```python
from build123d import *

# Parameters (mm, degrees)
SKETCH7_W               = 7.9375
SKETCH7_H               = 3.000000096
BOSS_EXTRUDE2_DEPTH     = 130.175
SKETCH8_W               = 3.000000096
SKETCH8_H               = 7.9375
BOSS_EXTRUDE3_DEPTH     = 130.175
BOSS_EXTRUDE4_DEPTH     = 130.175
CUT_EXTRUDE4_DEPTH      = 2.515570892
CUT_EXTRUDE4_DEPTH_BACK = 11.4775001
CUT_EXTRUDE5_DEPTH      = 11.4775001
CUT_EXTRUDE5_DEPTH_BACK = 2.500000148


with BuildPart() as part:
    # Sketch7 → Boss-Extrude2 (new body, symmetric)
    with BuildSketch(Plane.XY):
        with Locations((-6.50875, -3.000000096)):
            Rectangle(SKETCH7_W, SKETCH7_H)
    extrude(amount=BOSS_EXTRUDE2_DEPTH, both=True)

    # Sketch8 → Boss-Extrude3 (add, symmetric)
    with BuildSketch(Plane.XY):
        with Locations((-3.000000096, -6.50875)):
            Rectangle(SKETCH8_W, SKETCH8_H)
    extrude(amount=BOSS_EXTRUDE3_DEPTH, both=True)

    # Sketch11 → Boss-Extrude4 (add, symmetric)
    with BuildSketch(Plane.XY):
        with BuildLine():
            Line((-2.54, 1.500000048), (-2.54, -1.500000048))
            Line((-2.54, -1.500000048), (-10.4775, -1.500000048))
            Line((-10.4775, -1.500000048), (-10.4775, -4.500000144))
            Line((-10.4775, -4.500000144), (-6.745064174, -4.500000144))
            Line((-6.745064174, -4.500000144), (-4.500000144, -6.745064174))
            Line((-4.500000144, -6.745064174), (-4.500000144, -10.4775))
            Line((-4.500000144, -10.4775), (-1.500000048, -10.4775))
            Line((-1.500000048, -10.4775), (-1.500000048, -2.54))
            Line((-1.500000048, -2.54), (1.500000048, -2.54))
            add(Edge.make_bspline(
                [(-2.54, 1.500000048), (-1.295649087, 1.635512934), (-0.042467258, 0.473225958), (1.297713539, -0.292226779), (1.263724591, -2.340394541), (1.500000048, -2.54)],
                knots=[0, 0, 0, 0, 0.496686972, 0.741346965, 0.899739924, 0.899739924, 0.899739924, 0.899739924], degree=3))
        make_face()
    extrude(amount=BOSS_EXTRUDE4_DEPTH, both=True)

    # Sketch14 → Cut-Extrude4 (cut, two sides)
    with BuildSketch(Plane(origin=(0, 0, 0), x_dir=(1, 0, 0), z_dir=(0, 1, 0))) as cut_extrude4_sk:
        Polygon((-10.4775, -116.5225), (-10.4775, -137.4775), (10.4775, -137.4775), align=None)
        Polygon((-10.4775, 116.5225), (10.4775, 137.4775), (-10.4775, 137.4775), align=None)
    extrude(amount=CUT_EXTRUDE4_DEPTH, mode=Mode.SUBTRACT)
    extrude(cut_extrude4_sk.sketch, amount=-CUT_EXTRUDE4_DEPTH_BACK, mode=Mode.SUBTRACT)

    # Sketch17 → Cut-Extrude5 (cut, two sides)
    with BuildSketch(Plane(origin=(0, 0, 0), x_dir=(0, -1, 0), z_dir=(-1, 0, 0))) as cut_extrude5_sk:
        Polygon((10.4775, 137.4775), (10.4775, 116.5225), (-10.4775, 137.4775), align=None)
        Polygon((10.4775, -116.5225), (-10.4775, -137.4775), (10.4775, -137.4775), align=None)
    extrude(amount=CUT_EXTRUDE5_DEPTH, mode=Mode.SUBTRACT)
    extrude(cut_extrude5_sk.sketch, amount=-CUT_EXTRUDE5_DEPTH_BACK, mode=Mode.SUBTRACT)


solid = part.part
```
The listing builds one solid part. Answer for the finished solid, in the listing's coordinates (mm). A direction names the side the tool comes from. Round coordinates to 2 decimals unless told otherwise and drop trailing zeros. Answer as a JSON object with one key per item and string values. Group by question number.
Q1. Each of these flat-tipped pins is pushed along its axis until it touches: pin 1 Ø4 at (y, z) = (-5.5, -5.5) entering from +X; pin 2 Ø2 at (x, z) = (-7, 46) entering from -Y; pin 3 Ø4 at (x, z) = (-5, -50.5) entering from +Y. Where does it stop, or does it pass through?
Q2. Straight lines are drawn through the part: line 1 along Y through (x, z) = (0.75, 7.5); line 2 along Y through (x, z) = (-8.5, -36); line 3 along X through (y, z) = (-2.5, 59). For each, find the intervals that lie inside material, in ascending order.
Q3. Which of the six approach directions +Z, -Z, +X, -X, +Y, -Y give full straight-line access (tool end or side, diameter ignored) to faces 1 (the face through (-2, -6, -121)), 2 (the face through (-7, -1.5, 2)), 3 (the face through (-1.5, -7, 2))?
Check values:
{
 "1": {"pin 1": "x = -1.5", "pin 2": "y = -5.25", "pin 3": "y = -1.5"},
 "2": {"line 1": "-2.54 to -0.02", "line 2": "-4.5 to -1.5", "line 3": "-10.48 to 1.46"},
 "3": {"face 1": "-Z, +X, -X, -Y", "face 2": "+Z, -Z, -X, +Y", "face 3": "+Z, -Z, +X, -Y"}
}
